from build123d import *

# Parameters (mm, degrees)
F0_R     = 19.05
F1_DEPTH = 31.75
F2_DEPTH = 4.7625
F3_R     = 5.5626
F4_DEPTH = 4.7752
F5_DEPTH = 61.9262
F6_DEPTH = 61.9262


with BuildPart() as f1:
    # F0 (on Front) → F1 (new body, symmetric)
    with BuildSketch(Plane.XZ):
        with BuildLine():
            Line((70.111208, -4.7752), (-41.769909, -4.7752))
            ThreePointArc((-41.769909, -4.7752), (-69.341332, -40.856681), (-27.284214, -57.981385))
            ThreePointArc((-27.284214, -57.981385), (-16.552296, -46.789048), (-13.246168, -31.639394))
            Line((-13.246168, -31.639394), (-13.188227, -30.985492))
            ThreePointArc((-13.188227, -30.985492), (-10.131493, -24.800057), (-3.700401, -22.3012))
            Line((-3.700401, -22.3012), (47.719827, -22.3012))
            Line((47.719827, -22.3012), (70.111208, -22.3012))
            Line((70.111208, -22.3012), (70.111208, -4.7752))
        make_face()
        with Locations((-41.769909, -33.3502)):
            Circle(F0_R, mode=Mode.SUBTRACT)
    extrude(amount=F1_DEPTH, both=True)

    # F0 (on Front) → F2 (join, symmetric)
    with BuildSketch(Plane.XZ):
        with BuildLine():
            ThreePointArc((-13.246168, -31.639394), (-16.552296, -46.789048), (-27.284214, -57.981385))
            Line((-27.284214, -57.981385), (47.719827, -22.3012))
            Line((47.719827, -22.3012), (-3.700401, -22.3012))
            ThreePointArc((-3.700401, -22.3012), (-10.131493, -24.800057), (-13.188227, -30.985492))
            Line((-13.188227, -30.985492), (-13.246168, -31.639394))
        make_face()
    extrude(amount=F2_DEPTH, both=True)

    # F3 (on Top) → F4 (join)
    with BuildSketch(Plane.XY):
        with BuildLine():
            Line((11.361008, 19.05), (11.361008, -19.05))
            ThreePointArc((11.361008, -19.05), (15.080752, -28.030256), (24.061008, -31.75))
            ThreePointArc((24.061008, -31.75), (27.319684, -31.324813), (30.360163, -30.077721))
            Line((30.360163, -30.077721), (63.710363, -11.027721))
            ThreePointArc((63.710363, -11.027721), (68.395043, -6.375372), (70.111208, 0))
            ThreePointArc((70.111208, 0), (68.395043, 6.375372), (63.710363, 11.027721))
            Line((63.710363, 11.027721), (30.360163, 30.077721))
            ThreePointArc((30.360163, 30.077721), (27.319684, 31.324813), (24.061008, 31.75))
            ThreePointArc((24.061008, 31.75), (15.080752, 28.030256), (11.361008, 19.05))
        make_face()
        with Locations((24.061008, -19.05)):
            Circle(F3_R, mode=Mode.SUBTRACT)
        with Locations((24.061008, 19.05)):
            Circle(F3_R, mode=Mode.SUBTRACT)
        with Locations((57.411208, 0)):
            Circle(F3_R, mode=Mode.SUBTRACT)
    extrude(amount=-F4_DEPTH)

    # F3 (on Top) → F5 (cut, through all)
    with BuildSketch(Plane.XY):
        with Locations((24.061008, 19.05)):
            Circle(F3_R)
        with Locations((57.411208, 0)):
            Circle(F3_R)
        with Locations((24.061008, -19.05)):
            Circle(F3_R)
    extrude(amount=-F5_DEPTH, mode=Mode.SUBTRACT)

    # F3 (on Top) → F6 (cut, through all)
    with BuildSketch(Plane.XY):
        with BuildLine():
            ThreePointArc((30.360163, -30.077721), (27.319684, -31.324813), (24.061008, -31.75))
            Line((24.061008, -31.75), (70.111208, -31.75))
            Line((70.111208, -31.75), (70.111208, 0))
            ThreePointArc((70.111208, 0), (68.395043, -6.375372), (63.710363, -11.027721))
            Line((63.710363, -11.027721), (30.360163, -30.077721))
        make_face()
        with BuildLine():
            Line((70.111208, 31.75), (24.061008, 31.75))
            ThreePointArc((24.061008, 31.75), (27.319684, 31.324813), (30.360163, 30.077721))
            Line((30.360163, 30.077721), (63.710363, 11.027721))
            ThreePointArc((63.710363, 11.027721), (68.395043, 6.375372), (70.111208, 0))
            Line((70.111208, 0), (70.111208, 31.75))
        make_face()
    extrude(amount=-F6_DEPTH, mode=Mode.SUBTRACT)


solid = f1.part
Part model, mm, in its own coordinate system. A direction names the side the tool comes from. Give positions to 0.01 mm unless a question says otherwise; leave off trailing zeros. Write each loop counter-clockwise with the first axis right and the second up, starting at its lowest first coordinate (ties: lowest second). Pieces come first, ordered by that corner, then holes.
1) Cut at A-A on z = -20. Write the cut outline in (x, y).
Resolved:
outline: (-67.03, -31.75) - (-55.36, -31.75) - (-55.36, 31.75) - (-67.03, 31.75) - close; (-28.18, -31.75) - (24.06, -31.75) arc R12.7 ccw to (30.36, -30.08) - (63.71, -11.03) arc R12.7 ccw to (70.11, 0) arc R12.7 ccw to (63.71, 11.03) - (30.36, 30.08) arc R12.7 ccw to (24.06, 31.75) - (-28.18, 31.75) - close; hole circle Ø11.13 at (24.06, -19.05); hole circle Ø11.13 at (24.06, 19.05); hole circle Ø11.13 at (57.41, 0)
2) Probe L1, parallel to X at y = -10, z = -32.5; L2, parallel to X at y = -19, z = -16; L3, parallel to Z at x = 30.5, y = -19.5. List the from-to ranges inside material, lowest first.
Resolved:
L1: x = -70.33 to -60.8, -22.74 to -13.21
L2: x = -64.47 to -49.64, -33.9 to 18.5, 29.62 to 49.75
L3: z = -22.3 to 0
3) Two-plate mould, pull along Z, no slides. Class faces 1 (the face through (-10.204, 18.067, -24.867)), 2 (the face through (10, 4.762, -32)), 3 (the face through (-23.6, 0.44, -27.63)): released by +Z, released by -Z, zero draft, split by the parting line, or undercut.
Resolved:
face 1: released by -Z
face 2: zero draft
face 3: undercut
4) Cut at B-B on x = -55. Write the cut outline in (y, z), then the cut area to 3 significant figures.
Resolved:
outline: (-31.75, -58.68) - (31.75, -58.68) - (31.75, -47.06) - (-31.75, -47.06) - close; (-31.75, -19.64) - (31.75, -19.64) - (31.75, -8.02) - (-31.75, -8.02) - close
area: 1,480 mm2
5) Which spindle directions (+Z, -Z, +X, -X, +Y, -Y) get a long thin tool onto all of the face, cutting with end or side? Do faces 4 (the face through (10, -4.762, -32)), 5 (the face through (11.361, 0, -2)), 6 (the face through (15.18, 28.13, -2.35)). Say none if no direction does.
Resolved:
face 4: -Z, +X, -Y
face 5: +Z, -X, +Y, -Y
face 6: +Z, -X, +Y
6) Pin check, flat tips, straight feed: pin 1 (10.5 mm diameter, centred on x = 25, z = -37.5, fed in from -Y); pin 2 (6 mm diameter, centred on x = -32.5, y = -13, fed in from +Z); pin 3 (8 mm diameter, centred on y = -6, z = -43, fed in from -X); pin 4 (13 mm diameter, centred on x = 24.06, y = -19.05, fed in from +Z). Stop position of each tip, or through.
Resolved:
pin 1: stops at y = -4.76
pin 2: stops at z = -4.78
pin 3: stops at x = -69.78
pin 4: stops at z = 0
7) Cut at D-D on z = -7. Write the cut outline in (x, y).
Resolved:
outline: (-52.82, -31.75) - (24.06, -31.75) arc R12.7 ccw to (30.36, -30.08) - (63.71, -11.03) arc R12.7 ccw to (70.11, 0) arc R12.7 ccw to (63.71, 11.03) - (30.36, 30.08) arc R12.7 ccw to (24.06, 31.75) - (-52.82, 31.75) - close; hole circle Ø11.13 at (24.06, -19.05); hole circle Ø11.13 at (24.06, 19.05); hole circle Ø11.13 at (57.41, 0)
